```python
from build123d import *

# Parameters (mm, degrees)
CUT_EXTRUDE1_DEPTH      = 12
CUT_EXTRUDE1_DEPTH_BACK = 22
SKETCH3_R               = 3
CUT_EXTRUDE2_DEPTH      = 22
CUT_EXTRUDE2_DEPTH_BACK = 12


with BuildPart() as part:
    # Sketch1 → Revolve1 (revolve)
    with BuildSketch(Plane(origin=(0, 0, 0), x_dir=(0, 0, -1), z_dir=(1, 0, 0))):
        Polygon((21, 17.45), (7.03, 17.45), (7.03, 18.5), (0, 18.5), (0, 29), (-8, 29), (-8, 18.586235054), (-11, 16.803216346), (-11, 10), (21, 10), align=None)
    revolve(axis=Axis((0, 0, 11), (0, 0, -1)))

    # Sketch2 → Cut-Extrude1 (cut, two sides)
    with BuildSketch(Plane.XY) as cut_extrude1_sk:
        with BuildLine():
            Line((-2.55, -12.75), (2.55, -12.75))
            Line((2.55, -12.75), (2.55, -9.66941053))
            ThreePointArc((2.55, -9.66941053), (0, -10), (-2.55, -9.66941053))
            Line((-2.55, -9.66941053), (-2.55, -12.75))
        make_face()
    extrude(amount=CUT_EXTRUDE1_DEPTH, mode=Mode.SUBTRACT)
    extrude(cut_extrude1_sk.sketch, amount=-CUT_EXTRUDE1_DEPTH_BACK, mode=Mode.SUBTRACT)

    # Sketch3 → Cut-Extrude2 (cut, two sides)
    with BuildSketch(Plane(origin=(0, 0, 0), x_dir=(-1, 0, 0), z_dir=(0, 0, -1))) as cut_extrude2_sk:
        with Locations((-24, 0)):
            Circle(SKETCH3_R)
        with Locations((-12, 20.784609691)):
            Circle(SKETCH3_R)
        with Locations((12, 20.784609691)):
            Circle(SKETCH3_R)
        with Locations((24, 0)):
            Circle(SKETCH3_R)
        with Locations((12, -20.784609691)):
            Circle(SKETCH3_R)
        with Locations((-12, -20.784609691)):
            Circle(SKETCH3_R)
    extrude(amount=CUT_EXTRUDE2_DEPTH, mode=Mode.SUBTRACT)
    extrude(cut_extrude2_sk.sketch, amount=-CUT_EXTRUDE2_DEPTH_BACK, mode=Mode.SUBTRACT)


solid = part.part
```
Part model, mm, in its own coordinate system. A direction names the side the tool comes from. Give positions to 0.01 mm unless a question says otherwise; leave off trailing zeros. Write each loop counter-clockwise with the first axis right and the second up, starting at its lowest first coordinate (ties: lowest second). Pieces come first, ordered by that corner, then holes. Notation, with made-up numbers: M 80.25,-23 L 108.25,-23 A23 ccw 108.25,1 Z; hole C -31.75,-25.5 d2. An arc over 180 degrees is marked long. Use CSV: the item, a comma, the result in double quotes.
Item 1: Slice it at A-A on x = 0. Write the cut outline in (y, z), plus the area to 3 significant figures.
Taken from the geometry:
outline,"M -29,0 L -18.5,0 L -18.5,-7.03 L -17.45,-7.03 L -17.45,-21 L -12.75,-21 L -12.75,11 L -16.8,11 L -18.59,8 L -29,8 Z; M 10,-21 L 17.45,-21 L 17.45,-7.03 L 18.5,-7.03 L 18.5,0 L 29,0 L 29,8 L 18.59,8 L 16.8,11 L 10,11 Z"
area,"590 mm²"
Item 2: Drill centre lines: probe 1 along Y at (x, z) = (12, 4.5); probe 2 along Z at (x, y) = (-9.5, 26); probe 3 along Y at (x, z) = (3, -15). Where is each one in solid material? Low to high.
Taken from the geometry:
probe 1,"y = -26.4 to -23.78, -17.78 to 17.78, 23.78 to 26.4"
probe 2,"z = 0 to 8"
probe 3,"y = -17.19 to -9.54, 9.54 to 17.19"
Item 3: Slice it at B-B on z = -2.5. Write the cut outline in (x, y), plus the area to 3 significant figures.
Taken from the geometry:
outline,"C 0,0 d37; hole M -2.55,-12.75 L 2.55,-12.75 L 2.55,-9.67 A10 ccw long -2.55,-9.67 Z"
area,"746 mm²"
Item 4: Slice it at D-D on x = 22.5. Write the cut outline in (y, z), plus the area to 3 significant figures.
Taken from the geometry:
outline,"M -18.3,0 L -2.6,0 L -2.6,8 L -18.3,8 Z; M 2.6,0 L 18.3,0 L 18.3,8 L 2.6,8 Z"
area,"251 mm²"
Item 5: Which spindle directions (+Z, -Z, +X, -X, +Y, -Y) get a long thin tool onto all of the face, cutting with end or side? Do faces 1 (the face through (-19, 0, 8)), 2 (the face through (-7.2, 7.2, 11)), 3 (the face through (-2.55, -11, -5)), 4 (the face through (-14, 11, -7.03)). Say none if no direction does.
Taken from the geometry:
face 1,"+Z"
face 2,"+Z, +X, -X, +Y, -Y"
face 3,"+Z, -Z"
face 4,"-Z"
Item 6: Pull direction Y, two halves, no side cores. Call faces 5 (the face through (12.7, -23.7, 3.9)), 6 (the face through (-8, -8, -21)), 7 (the face through (-16.49, -3.66, 10.85)), 8 (the face through (-9.789, 22.812, 3.944)): +Y half, -Y half, draft (parallel to the pull), parting line (faces both ways), or undercut.
Taken from the geometry:
face 5,"undercut"
face 6,"draft"
face 7,"parting line"
face 8,"undercut"
Item 7: Slice it at C-C on y = 23. Write the cut outline in (x, z).
Taken from the geometry:
outline,"M -17.66,0 L -14.02,0 L -14.02,8 L -17.66,8 Z; M -9.98,0 L 9.98,0 L 9.98,8 L -9.98,8 Z; M 14.02,0 L 17.66,0 L 17.66,8 L 14.02,8 Z"
Item 8: Pin check, flat tips, straight feed: P1, Ø2.5, axis at y = -11, z = -9.5, coming from the -X side; P2, Ø8, axis at x = -24, y = 0, coming from the -Z side; P3, Ø2.5, axis at x = 0, z = -9.5, coming from the +Y side. Stop position of each tip, or through.
Taken from the geometry:
P1,"stops at x = -14.47"
P2,"stops at z = 0"
P3,"stops at y = 17.45"
